from build123d import *

# Parameters (mm, degrees)
SKETCH3_W                = 5
SKETCH3_H                = 30
BOSS_EXTRUDE1_DEPTH      = 5
SKETCH4_R                = 1.6
CUT_EXTRUDE1_DEPTH       = 75.540257579
BOSS_EXTRUDE2_REACH      = 75.485
BOSS_EXTRUDE2_END_RADIUS = 29
SKETCH5_W                = 2
SKETCH5_H                = 45
SKETCH5_W_2              = 45
SKETCH5_H_2              = 2
BOSS_EXTRUDE3_REACH      = 69.5
BOSS_EXTRUDE3_END_RADIUS = 29
SKETCH7_W                = 2
SKETCH7_H                = 3
CIRPATTERN1_COUNT        = 4


with BuildPart() as part:
    # Sketch2 → Revolve1 (revolve)
    with BuildSketch(Plane.XY):
        with BuildLine():
            Line((0, 29), (0, 30))
            ThreePointArc((0, 30), (21.213203436, 21.213203436), (30, 0))
            Line((30, 0), (29, 0))
            ThreePointArc((29, 0), (20.506096654, 20.506096654), (0, 29))
        make_face()
    revolve(axis=Axis((0, 0, 0), (0, 1, 0)))

    # Sketch3 → Boss-Extrude1 (add)
    with BuildSketch(Plane.XZ):
        with Locations((0, -45)):
            Rectangle(SKETCH3_W, SKETCH3_H)
        with BuildLine():
            Line((-2.5, -38), (2.5, -38))
            Line((2.5, -38), (12.22277757, -26.308006594))
            Line((12.22277757, -26.308006594), (12.219091313, -26.300072385))
            ThreePointArc((12.219091313, -26.300072385), (-0.967100454, -29.109666297), (-13.937737405, -25.431073041))
            Line((-13.937737405, -25.431073041), (-14.41834904, -26.308006594))
            Line((-14.41834904, -26.308006594), (-2.5, -38))
        make_face()
    extrude(amount=-BOSS_EXTRUDE1_DEPTH)

    # Sketch4 → Cut-Extrude1 (cut, through all)
    with BuildSketch(Plane(origin=(2.5, 0, 0), x_dir=(0, 0, -1), z_dir=(1, 0, 0))):
        with Locations((55, 2.5)):
            Circle(SKETCH4_R)
    extrude(amount=-CUT_EXTRUDE1_DEPTH, mode=Mode.SUBTRACT)

    # Boss-Extrude2: up to this sphere (the profile starts inside it)
    boss_extrude2_end = Location((0, 0, 0)) * Sphere(BOSS_EXTRUDE2_END_RADIUS, mode=Mode.PRIVATE)
    # Sketch5 → Boss-Extrude2 (add, up to the surface)
    with BuildSketch(Plane(origin=(0, 0, 0), x_dir=(1, 0, 0), z_dir=(0, 1, 0)), mode=Mode.PRIVATE) as boss_extrude2_sk1:
        Rectangle(SKETCH5_W, SKETCH5_H)
    boss_extrude2_tool1 = extrude(boss_extrude2_sk1.sketch, amount=BOSS_EXTRUDE2_REACH, mode=Mode.PRIVATE) & boss_extrude2_end
    add(boss_extrude2_tool1.solids().sort_by_distance((0, 0, 0))[0])
    # Sketch5 → Boss-Extrude2 (add, up to the surface)
    with BuildSketch(Plane(origin=(0, 0, 0), x_dir=(1, 0, 0), z_dir=(0, 1, 0)), mode=Mode.PRIVATE) as boss_extrude2_sk2:
        with Locations((0, -0.008687273)):
            Rectangle(SKETCH5_W_2, SKETCH5_H_2)
    boss_extrude2_tool2 = extrude(boss_extrude2_sk2.sketch, amount=BOSS_EXTRUDE2_REACH, mode=Mode.PRIVATE) & boss_extrude2_end
    add(boss_extrude2_tool2.solids().sort_by_distance((0, 0, 0.008687))[0])

    # Boss-Extrude3: up to this sphere (the profile starts inside it)
    boss_extrude3_end = Location((0, 0, 0)) * Sphere(BOSS_EXTRUDE3_END_RADIUS, mode=Mode.PRIVATE)
    # Sketch7 → Boss-Extrude3 (add, up to the surface)
    with BuildSketch(Plane(origin=(0, 0, -22.5), x_dir=(-1, 0, 0), z_dir=(0, 0, -1)), mode=Mode.PRIVATE) as boss_extrude3_sk1:
        with Locations((0, 1.5)):
            Rectangle(SKETCH7_W, SKETCH7_H)
    boss_extrude3_tool1 = extrude(boss_extrude3_sk1.sketch, amount=BOSS_EXTRUDE3_REACH, mode=Mode.PRIVATE) & boss_extrude3_end
    boss_extrude3 = boss_extrude3_tool1.solids().sort_by_distance((0, 1.5, -22.5))[0]
    add(boss_extrude3)

    # CirPattern1: Boss-Extrude3 ×4 about axis
    cirpattern1_axis = Axis((0, 0, 0), (0, 1, 0))
    for i in range(1, CIRPATTERN1_COUNT):
        add(boss_extrude3.rotate(cirpattern1_axis, i * 360 / CIRPATTERN1_COUNT))


solid = part.part
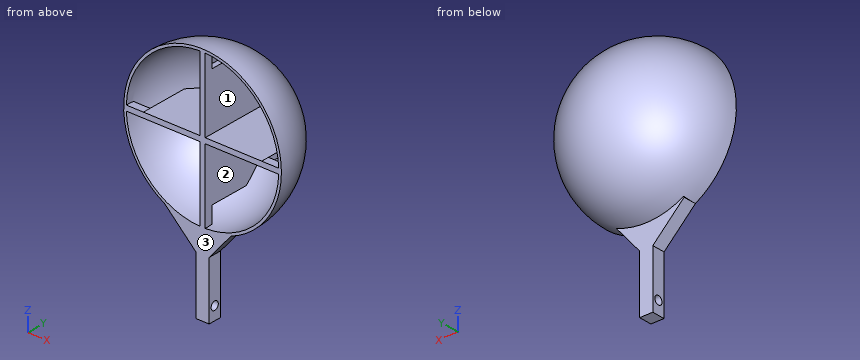
Here's how the part is built. I have some questions about the finished solid (model axes, mm). Face numbers are marked on the shaded views. Give positions to 0.01 mm unless a question says otherwise; leave off trailing zeros. Loops run counter-clockwise (first coordinate to the right, second up) from the corner with the lowest first, then second, coordinate; pieces in that order, holes last. Notation, with made-up numbers: (1, 35.25) -> (7, 35.25) arc R36 ccw to (7, 69.25) -> close; hole circle Ø2 at (46.5, 85). An arc over 180 degrees is marked (long way). Answer as a JSON object with one key per item and string values. Group by question number.
Item 1: Will these pins go through, and if not, where does the flat tip stop? pin 1 (13 mm diameter, centred on x = -2, z = -51, fed in from +Y); pin 2 (8 mm diameter, centred on y = 18, z = -15.5, fed in from -X); pin 3 (4 mm diameter, centred on y = 18.5, z = -3.5, fed in from -X).
Item 2: Imagine slicing it at A-A on z = -55. Write out the boundary of the cut face in (x, y), then the cut area to 3 significant figures.
Item 3: Imagine slicing it at D-D on x = -20. Write out the boundary of the cut face in (y, z).
Item 4: I need wall thicknesses on L1, parallel to Y at x = 1.2, z = -55; L2, parallel to Z at x = -12, y = 1; L3, parallel to Z at x = 22, y = 10.5. Which ranges of each line are inside material? Lowest first, please.
Item 5: Imagine slicing it at C-C on x = -26. Write out the boundary of the cut face in (y, z).
Item 6: Thinking about a two-plate mould opening in X: for the marked faces 1, 2 and 3, which applies, pulls with the +X half, pulls with the -X half, needs draft (parallel to the pull), parting line crosses it, or undercut?
Item 7: Imagine slicing it at B-B on y = 9. Write out the boundary of the cut face in (x, z), then the cut area to 3 significant figures.
Answer list:
{
 "1": {"pin 1": "stops at y = 5", "pin 2": "stops at x = -22.58", "pin 3": "stops at x = -24.84"},
 "2": {"outline": "(-2.5, 0) -> (2.5, 0) -> (2.5, 0.9) -> (-2.5, 0.9) -> close; (-2.5, 4.1) -> (2.5, 4.1) -> (2.5, 5) -> (-2.5, 5) -> close", "area": "9.00 mm2"},
 "3": {"outline": "(0, -22.36) arc R22.36 ccw to (0, 22.36) -> (0, 21) arc R21 cw to (20.98, 1.01) -> (0, 1.01) -> (0, -0.99) -> (20.98, -0.99) arc R21 cw to (0, -21) -> close"},
 "4": {"L1": "y = 0 to 0.9, 4.1 to 5", "L2": "z = -28.68 to -26.38, -0.99 to 1.01, 26.38 to 27.48", "L3": "z = -17.49 to -15.71, -0.99 to 1.01, 15.71 to 17.49"},
 "5": {"outline": "(0, -14.97) arc R14.97 ccw to (0, 14.97) -> (0, 12.85) arc R12.85 cw to (0, -12.85) -> close; (0, -1) -> (3, -1) -> (3, 1) -> (0, 1) -> close"},
 "6": {"face 1": "undercut", "face 2": "undercut", "face 3": "needs draft"},
 "7": {"outline": "circle Ø57.24 at (0, 0); (-22.5, -0.99) -> (-1, -0.99) -> (-1, -22.5) -> (1, -22.5) -> (1, -0.99) -> (22.5, -0.99) -> (22.5, 1.01) -> (1, 1.01) -> (1, 22.5) -> (-1, 22.5) -> (-1, 1.01) -> (-22.5, 1.01) -> close; hole circle Ø55.14 at (0, 0)", "area": "361 mm2"}
}
